Geometry: final body of the model. Coordinates: model frame, mm. A direction names the side the tool comes from. Round coordinates to 2 decimals unless told otherwise and drop trailing zeros. Order: outer loops, then holes, each group sorted by start corner. A loop starts at its lowest first (then second) coordinate and runs counter-clockwise, first axis right, second up. Notation, with made-up numbers: M 79,55.25 L 115,55.25 A14 ccw 115,80.25 Z; hole C 18.5,-39 d3. An arc over 180 degrees is marked long. Return JSON: item names as keys, results as strings. Group by question number.
Q1. Mould query, pull axis Y, two halves, no side actions, for faces 1 (the face through (9.897, -13.077, 28.755)), 2 (the face through (50, -13.5, 19.1)), 3 (the face through (19.1, 0, 36.5)). Classes: released by +Y, released by -Y, zero draft, split by the parting line, or undercut.
Q2. Contact query for flat-ended pins moving along their axis: pin 1 (20 mm diameter, centred on x = 25, z = 25, fed in from -Y); pin 2 (3 mm diameter, centred on x = 30.5, z = -7, fed in from +Y); pin 3 (1 mm diameter, centred on x = 31, y = -41, fed in from -Z); pin 4 (3 mm diameter, centred on x = 40, y = -41.5, fed in from +Z). Output: stop coordinate, or through.
Q3. Cut plane D-D on y = -42. Output: boundary loops of the cut face in (x, z), and give its area (3 significant figures).
Q4. Ray query, probe 1 along Z at (x, y) = (42.5, -25); probe 2 along Z at (x, y) = (32.75, -25). Return the intervals inside material, ascending.
Q5. Cut plane B-B on x = 17.5. Output: boundary loops of the cut face in (y, z).
Q6. Cut plane C-C on x = 41.5. Output: boundary loops of the cut face in (y, z), and give its area (3 significant figures).
Q7. Cut plane A-A on z = 25. Output: boundary loops of the cut face in (x, y), and give its area (3 significant figures).
Q8. Access query for faces 4 (the face through (40.45, -18.28, 35.54)), 5 (the face through (19.1, -13.5, 0)), 6 (the face through (19.1, -13.5, 50)). Directions: +Z, -Z, +X, -X, +Y, -Y. A direction counts if a zero-diameter tool reaches every point of the face in a straight line with its end or side. Return the directions, or none.
```python
from build123d import *

# Parameters (mm, degrees)
F0_W     = 50
F0_H     = 50
F1_DEPTH = 50
F2_R     = 12.5
F3_DEPTH = 25
F4_R     = 12.5
F5_DEPTH = 50
F6_R     = 12.5
F7_DEPTH = 50
F8_R     = 12.5
F9_DEPTH = 25


with BuildPart() as f1:
    # F0 (on Front) → F1 (new body)
    with BuildSketch(Plane.XZ):
        with Locations((25, 25)):
            Rectangle(F0_W, F0_H)
    extrude(amount=F1_DEPTH)

    # F2 (on face) → F3 (join)
    with BuildSketch(Plane.XY.offset(50)):
        with Locations((25, -25)):
            Circle(F2_R)
    extrude(amount=F3_DEPTH)

    # F4 (on face) → F5 (cut)
    with BuildSketch(Plane.YZ.offset(50)):
        with Locations((-25, 25)):
            Circle(F4_R)
    extrude(amount=-F5_DEPTH, mode=Mode.SUBTRACT)

    # F6 (on face) → F7 (cut)
    with BuildSketch(Plane.XZ.offset(50)):
        with Locations((25, 25)):
            Circle(F6_R)
    extrude(amount=-F7_DEPTH, mode=Mode.SUBTRACT)

    # F8 (on face) → F9 (join)
    with BuildSketch(Plane(origin=(0, 0, 0), x_dir=(1, 0, 0), z_dir=(0, 0, -1))):
        with Locations((25, 25)):
            Circle(F8_R)
    extrude(amount=F9_DEPTH)


solid = f1.part
```
Result sheet:
{
 "1": {"face 1": "undercut", "face 2": "zero draft", "face 3": "released by +Y"},
 "2": {"pin 1": "passes through", "pin 2": "stops at y = -13.16", "pin 3": "stops at z = 0", "pin 4": "stops at z = 50"},
 "3": {"outline": "M 0,0 L 50,0 L 50,50 L 0,50 Z; hole C 25,25 d25", "area": "2,010 mm²"},
 "4": {"probe 1": "z = 0 to 12.5, 37.5 to 50", "probe 2": "z = -25 to 12.5, 37.5 to 75"},
 "5": {"outline": "M -50,0 L -35,0 L -35,-25 L -15,-25 L -15,0 L 0,0 L 0,15 L -17.5,15 A12.5 cw -32.5,15 L -50,15 Z; M -50,35 L -32.5,35 A12.5 cw -17.5,35 L 0,35 L 0,50 L -15,50 L -15,75 L -35,75 L -35,50 L -50,50 Z"},
 "6": {"outline": "M -50,0 L 0,0 L 0,50 L -50,50 Z; hole C -25,25 d25", "area": "2,010 mm²"},
 "7": {"outline": "M 0,-50 L 12.5,-50 L 12.5,-37.5 L 0,-37.5 Z; M 0,-12.5 L 12.5,-12.5 L 12.5,0 L 0,0 Z; M 37.5,-50 L 50,-50 L 50,-37.5 L 37.5,-37.5 Z; M 37.5,-12.5 L 50,-12.5 L 50,0 L 37.5,0 Z", "area": "625 mm²"},
 "8": {"face 4": "+X, -X", "face 5": "-Z", "face 6": "+Z"}
}
